For this review, take the finished solid that the model builds, in its own axes (mm). Face numbers are marked on the shaded views. A direction names the side the tool comes from. Round coordinates to 2 decimals unless told otherwise and drop trailing zeros. Order: outer loops, then holes, each group sorted by start corner. A loop starts at its lowest first (then second) coordinate and runs counter-clockwise, first axis right, second up. Notation, with made-up numbers: M 25,29 L 84,29 A13 ccw 84,35 Z; hole C 78,12 d11. An arc over 180 degrees is marked long. Answer as a JSON object with one key per item and string values.
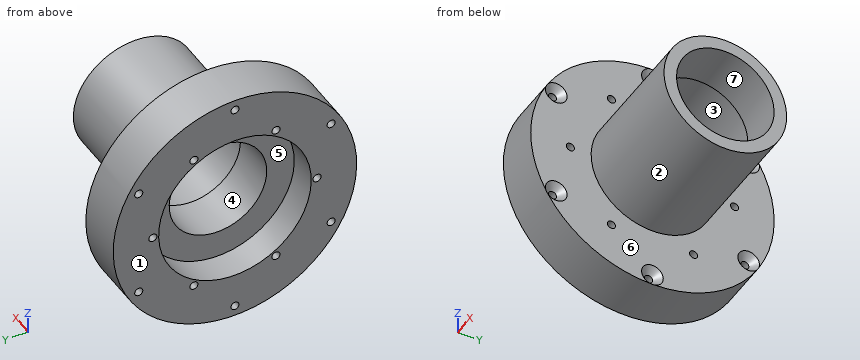
from build123d import *

# Parameters (mm, degrees)
F3_D           = 4.2
F3_CSINK_D     = 11.2
F3_CSINK_ANGLE = 90
F5_D           = 4.2


with BuildPart() as f1:
    # F0 (on Front) → F1 (revolve)
    with BuildSketch(Plane.XZ):
        Polygon((28, 25.25), (52, 25.25), (52, 31.75), (-14.5, 31.75), (-14.5, 63), (-39.5, 63), (-39.5, 39.5), (-24, 39.5), (-24, 25.25), (0, 25.25), (0, 26.25), (28, 26.25), align=None)
    revolve(axis=Axis((7.4011684002, 0, 0), (1, 0, 0)))

    # F3 (through all)
    with Locations(Plane.YZ.offset(-14.5)):
        with Locations((0, 57.5), (49.7964607176, 28.75), (49.7964607176, -28.75), (-49.7964607176, -28.75), (0, -57.5), (-49.7964607176, 28.75)):
            CounterSinkHole(F3_D / 2, F3_CSINK_D / 2, counter_sink_angle=F3_CSINK_ANGLE)

    # F5 (through all)
    with Locations(Plane.YZ.offset(-14.5)):
        with Locations((-21.25, 36.8060796608), (21.25, 36.8060796608), (42.5, 0), (21.25, -36.8060796608), (-21.25, -36.8060796608), (-42.5, 0)):
            Hole(F5_D / 2)


solid = f1.part
1) For L1, parallel to Z at x = -35, y = 0; L2, parallel to Z at x = -28, y = -21; L3, parallel to X at y = -30.5, z = -25.5, list the stretches that pass through material, from the lowest coordinate up.
Geometry check:
{"L1": "z = -63 to -59.6, -55.4 to -39.5, 39.5 to 55.4, 59.6 to 63", "L2": "z = -59.4 to -38.89, -34.72 to -33.46, 33.46 to 34.72, 38.89 to 59.4", "L3": "x = -39.5 to -14.5"}
2) Add section B-B on y = 42.5. State the section outline as (x, z) points.
Geometry check:
{"outline": "M -39.5,-46.51 L -14.5,-46.51 L -14.5,-2.1 L -39.5,-2.1 Z; M -39.5,2.1 L -14.5,2.1 L -14.5,46.51 L -39.5,46.51 Z"}
3) Add section C-C on z = 57.5. State the section outline as (x, y) points.
Geometry check:
{"outline": "M -39.5,-25.74 L -14.5,-25.74 L -14.5,-5.6 L -18,-2.1 L -39.5,-2.1 Z; M -39.5,2.1 L -18,2.1 L -14.5,5.6 L -14.5,25.74 L -39.5,25.74 Z"}
4) Machinability: for the marked faces 5, 6 and 7, which of the approach directions +Z, -Z, +X, -X, +Y, -Y give a long, thin tool a straight path to every point of the face, cutting with its end or side? Answer none if there is none.
Geometry check:
{"face 5": "-X", "face 6": "+X", "face 7": "+X, -X"}
5) Insertion check: P1, Ø5.5, axis at y = -49.8, z = -28.75, coming from the +X side; P2, Ø4, axis at x = 21.5, z = 3, coming from the -Y side; P3, Ø5.5, axis at y = 21.25, z = 36.81, coming from the +X side; P4, Ø4, axis at y = 0, z = 57.5, coming from the -X side. Each pin has a flat end and moves straight along its axis. Give the tip position at first contact, or say it passes through.
Geometry check:
{"P1": "stops at x = -17.35", "P2": "stops at y = -31.73", "P3": "stops at x = -14.5", "P4": "passes through"}
6) Add section D-D on x = 37.5. State the section outline as (y, z) points.
Geometry check:
{"outline": "C 0,0 d63.5; hole C 0,0 d50.5"}
7) Add section A-A on z = 0. State how many separate pieces and enclosed holes the cut face has, and give its area (3 significant figures).
Geometry check:
{"separate pieces": "4", "enclosed holes": "0", "area": "2,040 mm²"}
8) Mouldability with a two-part tool opening along Y and no side actions: class the marked faces 1, 2, 3 and 4 as +Y half, -Y half, draft (parallel to the pull), parting line (faces both ways), or undercut.
Geometry check:
{"face 1": "draft", "face 2": "parting line", "face 3": "undercut", "face 4": "undercut"}
